Can you work these out from the model? Positions are in its coordinate system, mm. A direction names the side the tool comes from. Give positions to 0.01 mm unless a question says otherwise; leave off trailing zeros. Loops run counter-clockwise (first coordinate to the right, second up) from the corner with the lowest first, then second, coordinate; pieces in that order, holes last. Notation, with made-up numbers: M 51.25,77 L 106.25,77 A23 cw 106.25,97 Z; hole C 62.25,37.5 d7. An arc over 180 degrees is marked long. Answer as a JSON object with one key per item and string values.
```python
from build123d import *

# Parameters (mm, degrees)
F0_R     = 8
F1_DEPTH = 17.5
F3_DEPTH = 25
F4_SIZE2 = 4
F4_SIZE  = 2
F6_R     = 8
F6_R_2   = 6.5
F7_DEPTH = 2


with BuildPart() as f1:
    # F0 (on Top) → F1 (new body, symmetric)
    with BuildSketch(Plane.XY):
        Circle(F0_R)
    extrude(amount=F1_DEPTH, both=True)

    # F2 (on face) → F3 (join)
    with BuildSketch(Plane.XY.offset(17.5)):
        with BuildLine():
            ThreePointArc((5, 6.2449979984), (0, 8), (-5, 6.2449979984))
            Line((-5, 6.2449979984), (-5, -6.2449979984))
            ThreePointArc((-5, -6.2449979984), (0, -8), (5, -6.2449979984))
            Line((5, -6.2449979984), (5, 6.2449979984))
        make_face()
    extrude(amount=F3_DEPTH)

    # F4
    f4_edges = [f1.edges().sort_by_distance(p)[0] for p in [
        (-5, 0, 42.5),
        (5, 0, 42.5),
    ]]
    f4_side = f1.faces().sort_by_distance((0, 0, 42.5))[0]
    chamfer(f4_edges, length=F4_SIZE, length2=F4_SIZE2, reference=f4_side)

    # F6 (on offset) → F7 (cut)
    with BuildSketch(Plane.XY.offset(26.5)):
        Circle(F6_R)
        Circle(F6_R_2, mode=Mode.SUBTRACT)
    extrude(amount=-F7_DEPTH, mode=Mode.SUBTRACT)


solid = f1.part
```
1) Please list where these lines run through material, in increasing order: line 1 along X through (y, z) = (-5.5, 30.5); line 2 along Y through (x, z) = (5, -11.5) (3 decimals); line 3 along Z through (x, y) = (-3.5, -6). Write a range as from..to.
Answer list:
{"line 1": "-5..5", "line 2": "-6.245..6.245", "line 3": "-17.5..24.5, 26.5..41.5"}
2) Suppose I cut it at A-A, the plane y = -5. Write out the boundary of the cut face in (x, z) (3 decimals).
Answer list:
{"outline": "M -6.245,-17.5 L 6.245,-17.5 L 6.245,17.5 L 5,17.5 L 5,24.5 L 4.153,24.5 L 4.153,26.5 L 5,26.5 L 5,38.5 L 3,42.5 L -3,42.5 L -5,38.5 L -5,26.5 L -4.153,26.5 L -4.153,24.5 L -5,24.5 L -5,17.5 L -6.245,17.5 Z"}
3) Suppose I cut it at D-D, the plane y = 0. Write out the boundary of the cut face in (x, z), and give its area (3 significant figures).
Answer list:
{"outline": "M -8,-17.5 L 8,-17.5 L 8,17.5 L 5,17.5 L 5,38.5 L 3,42.5 L -3,42.5 L -5,38.5 L -5,17.5 L -8,17.5 Z", "area": "802 mm^2"}
4) If we mould it in two halves opening along Z, with no side actions, what happens to faces 6 (the flat face through (5, 0, 28)), 7 (the flat face through (0, 7, 26.5)), 8 (the flat face through (0, -7, 26.5)), 9 (the flat face through (6, 0, 17.5))? For each: +Z half, -Z half, draft (parallel to the pull), parting line (faces both ways), or undercut.
Answer list:
{"face 6": "draft", "face 7": "undercut", "face 8": "undercut", "face 9": "+Z half"}
5) Will these pins go through, and if not, where does the flat tip stop? pin 1 Ø6 at (y, z) = (-1.5, 23) entering from -X; pin 2 Ø1.5 at (x, z) = (-4.5, 27.5) entering from -Y; pin 3 Ø0.9 at (x, y) = (-6, 2) entering from +Z.
Answer list:
{"pin 1": "x = -5", "pin 2": "y = -7.07", "pin 3": "z = 17.5"}
6) Suppose I cut it at C-C, the plane x = -1.75. Write out the boundary of the cut face in (y, z), and give its area (3 significant figures).
Answer list:
{"outline": "M -7.81,-17.5 L 7.81,-17.5 L 7.81,24.5 L 6.26,24.5 L 6.26,26.5 L 7.81,26.5 L 7.81,42.5 L -7.81,42.5 L -7.81,26.5 L -6.26,26.5 L -6.26,24.5 L -7.81,24.5 Z", "area": "931 mm^2"}
7) Suppose I cut it at B-B, the plane z = 30.5. Write out the boundary of the cut face in (x, y) (3 decimals), and give its area (3 significant figures).
Answer list:
{"outline": "M -5,-6.245 A8 ccw 5,-6.245 L 5,6.245 A8 ccw -5,6.245 Z", "area": "149 mm^2"}
8) For faces 1 (the flat face through (0, 7, 24.5)), 2 (the cylindrical face through (-0.1, -6.5, 25.5)), 3 (the flat face through (0, 0, 42.5)), 4 (the cylindrical face through (0, 8, 34)), 5 (the flat face through (-6, 0, 17.5)), which set-ups out of +Z, -Z, +X, -X, +Y, -Y let a thin tool reach every point of the face, with its end or its side?
Answer list:
{"face 1": "+Y", "face 2": "-Y", "face 3": "+Z, +X, -X, +Y, -Y", "face 4": "+Z, -Z, +Y", "face 5": "+Z, -X, +Y, -Y"}
